```python
from build123d import *
from build123d.topology import SkipClean

# Parameters (mm, degrees)
EXTRUDE_1_DEPTH                 = 2.5
SKETCH_6_R                      = 2
CUT_EXTRUDE_1_DEPTH             = 3
EXTRUDE_2_DEPTH                 = 2.5
CUT_EXTRUDE_2_DEPTH             = 1
SKETCH_8_R                      = 4
SKETCH_8_R_2                    = 1
CUT_EXTRUDE_3_DEPTH             = 1.5
SKETCH_9_R                      = 2
CUT_EXTRUDE_4_DEPTH             = 2.5
CUT_EXTRUDE_5_DEPTH             = 1
SKETCH_11_R                     = 4
SKETCH_11_R_2                   = 1
CUT_EXTRUDE_6_DEPTH             = 1.5
EXTRUDE_3_REACH                 = 101.914
SKETCH_12_W                     = 36
SKETCH_12_H                     = 2.5
EXTRUDE_3_DIRECTION_2_REACH     = 101.914
CUT_EXTRUDE_7_REACH             = 108.035
SKETCH_13_W                     = 9
SKETCH_13_H                     = 27
SKETCH_13_H_2                   = 11
SKETCH_13_H_3                   = 11.890625
CUT_EXTRUDE_8_REACH             = 108.035
SKETCH_14_W                     = 9
SKETCH_14_H                     = 27
SKETCH_14_H_2                   = 11
SKETCH_14_H_3                   = 11.890625
CUT_EXTRUDE_8_DIRECTION_2_DEPTH = 107.035371457
CUT_EXTRUDE_9_DEPTH             = 57.857277459
CUT_EXTRUDE_9_DEPTH_BACK        = 57.857277459
SKETCH_15_W                     = 30
SKETCH_15_H                     = 9
FILLET_1_R                      = 1


with BuildPart() as part:
    # Sketch 4 → Extrude 1 (new body)
    with BuildSketch(Plane.ZY.offset(18)):
        with BuildLine():
            Line((-7.5, 90), (-7.5, 0))
            ThreePointArc((-7.5, 0), (0, -7.5), (7.5, 0))
            Line((7.5, 0), (7.5, 90))
            ThreePointArc((7.5, 90), (0, 97.5), (-7.5, 90))
        make_face()
    extrude(amount=EXTRUDE_1_DEPTH)

    # Sketch 6 → Cut-Extrude 1 (cut)
    with BuildSketch(Plane.ZY.offset(20.5)):
        Circle(SKETCH_6_R)
    extrude(amount=-CUT_EXTRUDE_1_DEPTH, mode=Mode.SUBTRACT)

    # Sketch 10 → Cut-Extrude 5 (cut)
    with BuildSketch(Plane.ZY.offset(20.5)):
        with BuildLine():
            Line((-2.75, 73), (-3.6, 88.256440423))
            ThreePointArc((-3.6, 88.256440423), (0, 94), (3.6, 88.256440423))
            Line((3.6, 88.256440423), (2.75, 73))
            ThreePointArc((2.75, 73), (0, 71), (-2.75, 73))
        make_face()
    extrude(amount=-CUT_EXTRUDE_5_DEPTH, mode=Mode.SUBTRACT)

    # Sketch 11 → Cut-Extrude 6 (cut)
    with SkipClean():  # the faces are left unmerged after this step: merging them gives an invalid solid
        with BuildSketch(Plane.ZY.offset(19.5)):
            with Locations((0, 90)):
                Circle(SKETCH_11_R)
            with Locations((0, 74.05)):
                Circle(SKETCH_11_R_2)
            with Locations((0, 81.55)):
                Circle(SKETCH_11_R_2)
        extrude(amount=-CUT_EXTRUDE_6_DEPTH, mode=Mode.SUBTRACT)

    # Extrude 3: up to this face of the body (flat: up to its plane)
    extrude_3_end = Plane(part.part.faces().sort_by_distance((-19.25, 45, 7.5))[0])
    # Sketch 12 → Extrude 3 (add, up to the picked face)
    with BuildSketch(Plane.XY, mode=Mode.PRIVATE) as extrude_3_sk1:
        with Locations((0, 53.75)):
            Rectangle(SKETCH_12_W, SKETCH_12_H)
    extrude_3_tool1 = split(extrude(extrude_3_sk1.sketch, amount=EXTRUDE_3_REACH, mode=Mode.PRIVATE), bisect_by=extrude_3_end, keep=Keep.BOTH, mode=Mode.PRIVATE)
    # Sketch 12 → Extrude 3 (add, up to the picked face)
    with BuildSketch(Plane.XY, mode=Mode.PRIVATE) as extrude_3_sk2:
        with Locations((0, 36.25)):
            Rectangle(SKETCH_12_W, SKETCH_12_H)
    extrude_3_tool2 = split(extrude(extrude_3_sk2.sketch, amount=EXTRUDE_3_REACH, mode=Mode.PRIVATE), bisect_by=extrude_3_end, keep=Keep.BOTH, mode=Mode.PRIVATE)


with BuildPart() as body_2:
    # Sketch 5 → Extrude 2 (new body)
    with BuildSketch(Plane(origin=(18, 0, 0), x_dir=(0, 0, -1), z_dir=(1, 0, 0))):
        with BuildLine():
            Line((-7.5, 0), (-7.5, 90))
            ThreePointArc((-7.5, 90), (0, 97.5), (7.5, 90))
            Line((7.5, 90), (7.5, 0))
            ThreePointArc((7.5, 0), (0, -7.5), (-7.5, 0))
        make_face()
    extrude(amount=EXTRUDE_2_DEPTH)

    # Sketch 7 → Cut-Extrude 2 (cut)
    with BuildSketch(Plane(origin=(20.5, 0, 0), x_dir=(0, 0, -1), z_dir=(1, 0, 0))):
        with BuildLine():
            Line((-3.6, 1.743559577), (-2.75, 17))
            ThreePointArc((-2.75, 17), (0, 19), (2.75, 17))
            Line((2.75, 17), (3.6, 1.743559577))
            ThreePointArc((3.6, 1.743559577), (0, -4), (-3.6, 1.743559577))
        make_face()
    extrude(amount=-CUT_EXTRUDE_2_DEPTH, mode=Mode.SUBTRACT)

    # Sketch 8 → Cut-Extrude 3 (cut)
    with SkipClean():  # the faces are left unmerged after this step: merging them gives an invalid solid
        with BuildSketch(Plane(origin=(19.5, 0, 0), x_dir=(0, 0, -1), z_dir=(1, 0, 0))):
            Circle(SKETCH_8_R)
            with Locations((0, 15.95)):
                Circle(SKETCH_8_R_2)
            with Locations((0, 8.45)):
                Circle(SKETCH_8_R_2)
        extrude(amount=-CUT_EXTRUDE_3_DEPTH, mode=Mode.SUBTRACT)

    # Sketch 9 → Cut-Extrude 4 (cut)
    with SkipClean():  # the faces are left unmerged after this step: merging them gives an invalid solid
        with BuildSketch(Plane(origin=(20.5, 0, 0), x_dir=(0, 0, -1), z_dir=(1, 0, 0))):
            with Locations((0, 90)):
                Circle(SKETCH_9_R)
        extrude(amount=-CUT_EXTRUDE_4_DEPTH, mode=Mode.SUBTRACT)


with BuildPart() as part_1:
    add(part.part)

    add(body_2.part)  # Extrude 3 merges body 2
    add(extrude_3_tool1.solids().sort_by(Axis((0, 53.75, 0), (0, 0, 1)))[0])
    add(extrude_3_tool2.solids().sort_by(Axis((0, 36.25, 0), (0, 0, 1)))[0])

    # Extrude 3 direction 2: up to this face of the body (flat: up to its plane)
    extrude_3_direction_2_end = Plane(part_1.part.faces().sort_by_distance((-19.25, 45, -7.5))[0])
    # Sketch 12 → Extrude 3 direction 2 (add, up to the picked face)
    with BuildSketch(Plane.XY, mode=Mode.PRIVATE) as extrude_3_direction_2_sk1:
        with Locations((0, 53.75)):
            Rectangle(SKETCH_12_W, SKETCH_12_H)
    extrude_3_direction_2_tool1 = split(extrude(extrude_3_direction_2_sk1.sketch, amount=-EXTRUDE_3_DIRECTION_2_REACH, mode=Mode.PRIVATE), bisect_by=extrude_3_direction_2_end, keep=Keep.BOTH, mode=Mode.PRIVATE)
    # Sketch 12 → Extrude 3 direction 2 (add, up to the picked face)
    with BuildSketch(Plane.XY, mode=Mode.PRIVATE) as extrude_3_direction_2_sk2:
        with Locations((0, 36.25)):
            Rectangle(SKETCH_12_W, SKETCH_12_H)
    extrude_3_direction_2_tool2 = split(extrude(extrude_3_direction_2_sk2.sketch, amount=-EXTRUDE_3_DIRECTION_2_REACH, mode=Mode.PRIVATE), bisect_by=extrude_3_direction_2_end, keep=Keep.BOTH, mode=Mode.PRIVATE)
    add(extrude_3_direction_2_tool1.solids().sort_by(Axis((0, 53.75, 0), (0, 0, -1)))[0])
    add(extrude_3_direction_2_tool2.solids().sort_by(Axis((0, 36.25, 0), (0, 0, -1)))[0])

    # Sketch 13 → Cut-Extrude 7 (cut, up to next)
    with BuildSketch(Plane.ZY.offset(20.5), mode=Mode.PRIVATE) as cut_extrude_7_sk1:
        with Locations((0, 19.5)):
            Rectangle(SKETCH_13_W, SKETCH_13_H)
    cut_extrude_7_tool1 = extrude(cut_extrude_7_sk1.sketch, amount=-CUT_EXTRUDE_7_REACH, mode=Mode.PRIVATE) & part_1.part
    # Sketch 13 → Cut-Extrude 7 (cut, up to next)
    with BuildSketch(Plane.ZY.offset(20.5), mode=Mode.PRIVATE) as cut_extrude_7_sk2:
        with Locations((0, 45)):
            Rectangle(SKETCH_13_W, SKETCH_13_H_2)
    cut_extrude_7_tool2 = extrude(cut_extrude_7_sk2.sketch, amount=-CUT_EXTRUDE_7_REACH, mode=Mode.PRIVATE) & part_1.part
    # Sketch 13 → Cut-Extrude 7 (cut, up to next)
    with BuildSketch(Plane.ZY.offset(20.5), mode=Mode.PRIVATE) as cut_extrude_7_sk3:
        with Locations((0, 62.9453125)):
            Rectangle(SKETCH_13_W, SKETCH_13_H_3)
    cut_extrude_7_tool3 = extrude(cut_extrude_7_sk3.sketch, amount=-CUT_EXTRUDE_7_REACH, mode=Mode.PRIVATE) & part_1.part
    add(cut_extrude_7_tool1.solids().sort_by_distance((-20.5, 19.5, 0))[0], mode=Mode.SUBTRACT)
    add(cut_extrude_7_tool2.solids().sort_by_distance((-20.5, 45, 0))[0], mode=Mode.SUBTRACT)
    add(cut_extrude_7_tool3.solids().sort_by_distance((-20.5, 62.945312, 0))[0], mode=Mode.SUBTRACT)

    # Sketch 14 → Cut-Extrude 8 (cut, up to next)
    with BuildSketch(Plane(origin=(20.5, 0, 0), x_dir=(0, 0, -1), z_dir=(1, 0, 0)), mode=Mode.PRIVATE) as cut_extrude_8_sk1:
        with Locations((0, 70.5)):
            Rectangle(SKETCH_14_W, SKETCH_14_H)
    cut_extrude_8_tool1 = extrude(cut_extrude_8_sk1.sketch, amount=-CUT_EXTRUDE_8_REACH, mode=Mode.PRIVATE) & part_1.part
    # Sketch 14 → Cut-Extrude 8 (cut, up to next)
    with BuildSketch(Plane(origin=(20.5, 0, 0), x_dir=(0, 0, -1), z_dir=(1, 0, 0)), mode=Mode.PRIVATE) as cut_extrude_8_sk2:
        with Locations((0, 45)):
            Rectangle(SKETCH_14_W, SKETCH_14_H_2)
    cut_extrude_8_tool2 = extrude(cut_extrude_8_sk2.sketch, amount=-CUT_EXTRUDE_8_REACH, mode=Mode.PRIVATE) & part_1.part
    # Sketch 14 → Cut-Extrude 8 (cut, up to next)
    with BuildSketch(Plane(origin=(20.5, 0, 0), x_dir=(0, 0, -1), z_dir=(1, 0, 0)), mode=Mode.PRIVATE) as cut_extrude_8_sk3:
        with Locations((0, 27.0546875)):
            Rectangle(SKETCH_14_W, SKETCH_14_H_3)
    cut_extrude_8_tool3 = extrude(cut_extrude_8_sk3.sketch, amount=-CUT_EXTRUDE_8_REACH, mode=Mode.PRIVATE) & part_1.part
    add(cut_extrude_8_tool1.solids().sort_by_distance((20.5, 70.5, 0))[0], mode=Mode.SUBTRACT)
    add(cut_extrude_8_tool2.solids().sort_by_distance((20.5, 45, 0))[0], mode=Mode.SUBTRACT)
    add(cut_extrude_8_tool3.solids().sort_by_distance((20.5, 27.054688, 0))[0], mode=Mode.SUBTRACT)

    # Sketch 14 → Cut-Extrude 8 direction 2 (cut)
    with SkipClean():  # the faces are left unmerged after this step: merging them gives an invalid solid
        with BuildSketch(Plane(origin=(20.5, 0, 0), x_dir=(0, 0, -1), z_dir=(1, 0, 0))):
            with Locations((0, 70.5)):
                Rectangle(SKETCH_14_W, SKETCH_14_H)
            with Locations((0, 45)):
                Rectangle(SKETCH_14_W, SKETCH_14_H_2)
            with Locations((0, 27.0546875)):
                Rectangle(SKETCH_14_W, SKETCH_14_H_3)
        extrude(amount=CUT_EXTRUDE_8_DIRECTION_2_DEPTH, mode=Mode.SUBTRACT)

    # Sketch 15 → Cut-Extrude 9 (cut, two sides: drawn at the far end of the back side and taken through both)
    with SkipClean():  # the faces are left unmerged after this step: merging them gives an invalid solid
        with BuildSketch(Plane(origin=(0, 45, 0), x_dir=(1, 0, 0), z_dir=(0, 1, 0)).offset(-CUT_EXTRUDE_9_DEPTH_BACK)):
            Rectangle(SKETCH_15_W, SKETCH_15_H)
        extrude(amount=CUT_EXTRUDE_9_DEPTH + CUT_EXTRUDE_9_DEPTH_BACK, mode=Mode.SUBTRACT)

    # Fillet 1
    fillet_1_edges = [part_1.edges().sort_by_distance(p)[0] for p in [
        (-19.25, 33, -4.5),
        (-19.25, 6, -4.5),
        (-19.25, 6, 4.5),
        (-19.25, 33, 4.5),
        (-19.25, 50.5, -4.5),
        (-19.25, 39.5, -4.5),
        (-19.25, 39.5, 4.5),
        (-19.25, 50.5, 4.5),
        (19.25, 50.5, 4.5),
        (19.25, 39.5, 4.5),
        (19.25, 39.5, -4.5),
        (19.25, 50.5, -4.5),
        (-15, 53.75, 4.5),
        (-15, 36.25, 4.5),
        (-15, 53.75, -4.5),
        (-15, 36.25, -4.5),
        (15, 53.75, -4.5),
        (15, 36.25, -4.5),
        (15, 53.75, 4.5),
        (15, 36.25, 4.5),
        (-18, 52.5, -3.75),
        (-18, 55, -3.75),
        (18, 55, 3.75),
        (18, 52.5, 3.75),
        (18, 37.5, 3.75),
        (18, 35, 3.75),
        (-18, 35, -3.75),
        (-18, 37.5, -3.75),
    ]]
    fillet(fillet_1_edges, radius=FILLET_1_R)


solid = part_1.part
```
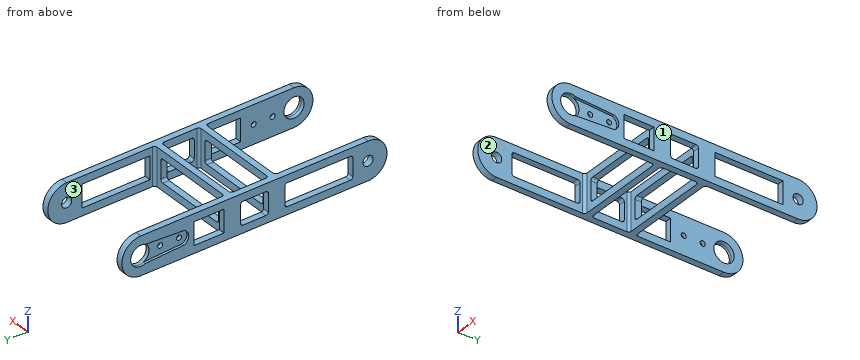
Source: CAD feature listing. Evaluate the final solid. Frame: model axes, mm. Face numbers are marked on the shaded views. A direction names the side the tool comes from. Round coordinates to 2 decimals unless told otherwise and drop trailing zeros. Loops run counter-clockwise (first coordinate to the right, second up) from the corner with the lowest first, then second, coordinate; pieces in that order, holes last. Notation, with made-up numbers: M 80,-31.5 L 102,-31.5 A16 cw 102,-7.5 Z; hole C 4.25,76.25 d6. An arc over 180 degrees is marked long. Use a Markdown table: item, result. Add a question column.
1. Section query B-B on x = 1. Return the cut outline in (y, z).
2. Section query C-C on z = 6.5. Return the cut outline in (x, y).
3. Section query A-A on y = 46. Return the cut outline in (x, z).
4. Reachability of the marked faces 1, 2 and 3 from +Z, -Z, +X, -X, +Y, -Y: full face, straight path, thin tool, end or side. Return the list, or none.
5. Section query D-D on z = 0. Give the number of separate pieces and of enclosed holes in the cut face, then the cut area to 3 significant figures.
6. Contact query for flat-ended pins moving along their axis: P1, Ø3.5, axis at y = 7.5, z = -0.5, coming from the +X side; P2, Ø7.5, axis at x = 0.5, z = 2.5, coming from the -Y side; P3, Ø7.5, axis at x = 5.5, z = 2, coming from the +Y side. Output: stop coordinate, or through.
7. Line query: line 1 (X direction, y = 85, z = 6); line 2 (Y direction, x = -6, z = 5.75); line 3 (Z direction, x = 19, y = 0). Output: solid intervals per line, ascending.
Reported:
| question | item | result |
|---|---|---|
| 1 | outline | M 35,-7.5 L 37.5,-7.5 L 37.5,-4.5 L 35,-4.5 Z; M 35,4.5 L 37.5,4.5 L 37.5,7.5 L 35,7.5 Z; M 52.5,-7.5 L 55,-7.5 L 55,-4.5 L 52.5,-4.5 Z; M 52.5,4.5 L 55,4.5 L 55,7.5 L 52.5,7.5 Z |
| 2 | outline | M -20.5,-3.74 L -18,-3.74 L -18,34 A1 cw -17,35 L 17,35 A1 cw 18,34 L 18,-3.74 L 20.5,-3.74 L 20.5,93.74 L 18,93.74 L 18,56 A1 cw 17,55 L -17,55 A1 cw -18,56 L -18,93.74 L -20.5,93.74 Z; hole M -18,38.5 A1 ccw -17,37.5 L 17,37.5 A1 ccw 18,38.5 L 18,51.5 A1 ccw 17,52.5 L -17,52.5 A1 ccw -18,51.5 Z |
| 3 | outline | M -20.5,-7.5 L -18,-7.5 L -18,-4.5 L -20.5,-4.5 Z; M -20.5,4.5 L -18,4.5 L -18,7.5 L -20.5,7.5 Z; M 18,-7.5 L 20.5,-7.5 L 20.5,-4.5 L 18,-4.5 Z; M 18,4.5 L 20.5,4.5 L 20.5,7.5 L 18,7.5 Z |
| 4 | face 1 | +Z, -Z, +X, +Y, -Y |
| 4 | face 2 | +Z, -Z, -Y |
| 4 | face 3 | +Z, -Z, +Y |
| 5 | separate pieces | 16 |
| 5 | enclosed holes | 0 |
| 5 | area | 205 mm² |
| 6 | P1 | stops at x = 19.5 |
| 6 | P2 | stops at y = 35 |
| 6 | P3 | stops at y = 55 |
| 7 | line 1 | x = -20.5 to -18, 18 to 20.5 |
| 7 | line 2 | y = 35 to 37.5, 52.5 to 55 |
| 7 | line 3 | z = -7.5 to -4, 4 to 7.5 |
